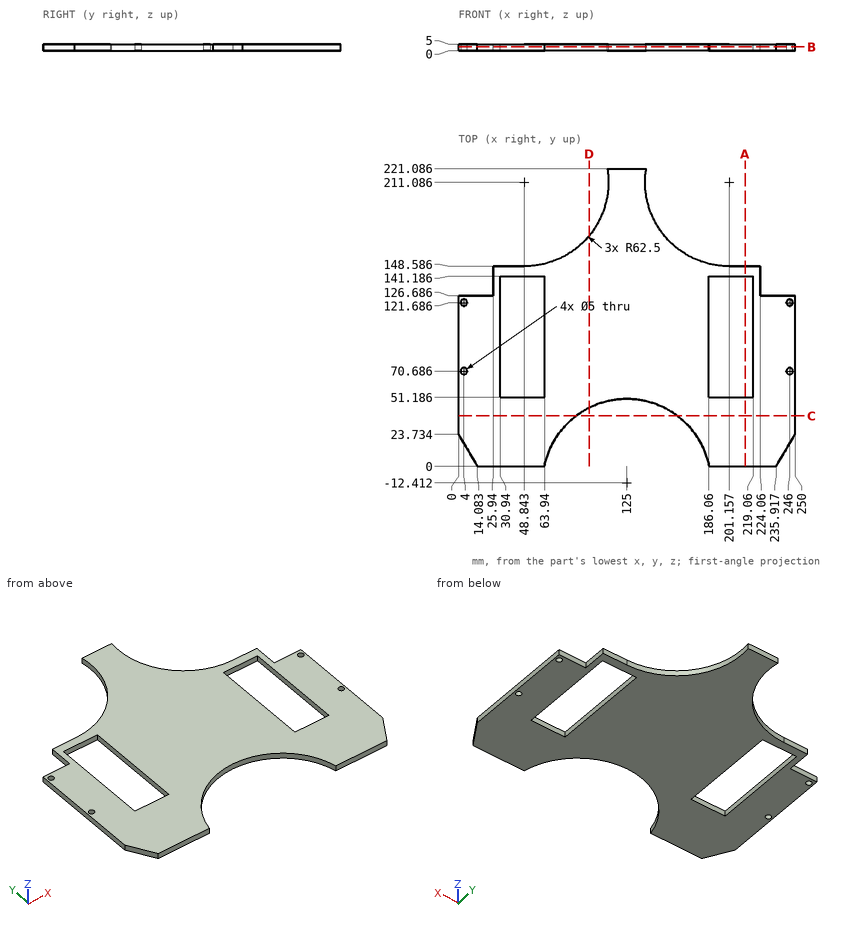
The figure shows three views and two pictorial views of one solid part (mm, origin at its lowest corner). Answer the questions. Coordinates: 2 decimals unless noted, no trailing zeros. Loops run counter-clockwise (first coordinate to the right, second up) from the corner with the lowest first, then second, coordinate; pieces in that order, holes last. Notation, with made-up numbers: (58.25, 70.25) - (94.25, 70.25) arc R17 ccw to (94.25, 95.25) - close; hole circle Ø7 at (-39.75, -33). An arc over 180 degrees is marked (long way). Answer in a Markdown table with one row per item.
Q1. Find section A-A on x = 213. Write down the section's boundary in (y, z) (1 decimal).
Here are the results:
| item | result |
|---|---|
| outline | (0, 0) - (51.2, 0) - (51.2, 5) - (0, 5) - close; (141.2, 0) - (148.6, 0) - (148.6, 5) - (141.2, 5) - close |
Q2. Find section C-C on y = 37.5. Write down the section's boundary in (x, z).
Here are the results:
| item | result |
|---|---|
| outline | (0, 0) - (87.38, 0) - (87.38, 5) - (0, 5) - close; (162.62, 0) - (250, 0) - (250, 5) - (162.62, 5) - close |
Q3. Straight lines are drawn through the part: line 1 along X through (y, z) = (65, 0.9); line 2 along X through (y, z) = (139.5, 2.8); line 3 along Y through (x, z) = (246, 2.1) (1 decimal). For each, find the intervals that lie inside material, in ascending order. Write a range as [from, to].
Here are the results:
| item | result |
|---|---|
| line 1 | x = [0, 30.94], [63.94, 186.06], [219.06, 250] |
| line 2 | x = [25.94, 30.94], [63.94, 186.06], [219.06, 224.06] |
| line 3 | y = [17, 68.2], [73.2, 119.2], [124.2, 126.7] |
Q4. Find section D-D on x = 97. Write down the section's boundary in (y, z) (1 decimal), plus the area to 3 significant figures.
Here are the results:
| item | result |
|---|---|
| outline | (43.5, 0) - (171.2, 0) - (171.2, 5) - (43.5, 5) - close |
| area | 639 mm^2 |
Q5. Find section B-B on z = 2.95. Write down the section's boundary in (x, y) (1 decimal).
Here are the results:
| item | result |
|---|---|
| outline | (0, 23.7) - (14.1, 0) - (63.7, 0) arc R62.5 cw to (186.3, 0) - (235.9, 0) - (250, 23.7) - (250, 126.7) - (224.1, 126.7) - (224.1, 148.6) - (201.2, 148.6) arc R62.5 cw to (139.5, 221.1) - (110.5, 221.1) arc R62.5 cw to (48.8, 148.6) - (25.9, 148.6) - (25.9, 126.7) - (0, 126.7) - close; hole circle Ø5 at (4, 70.7); hole circle Ø5 at (4, 121.7); hole (30.9, 51.2) - (63.9, 51.2) - (63.9, 141.2) - (30.9, 141.2) - close; hole (186.1, 51.2) - (219.1, 51.2) - (219.1, 141.2) - (186.1, 141.2) - close; hole circle Ø5 at (246, 70.7); hole circle Ø5 at (246, 121.7) |
Q6. Given P1, Ø1.5, axis at x = 196, z = 3, coming from the +Y side (1 decimal); P2, Ø1.5, axis at x = 101.5, z = 2.5, coming from the +Y side; P3, Ø3, axis at x = 62, z = 4, coming from the +Y side, each flat-ended and moving along its own axis, determine where each tip first touches the part or whether it passes through.
Here are the results:
| item | result |
|---|---|
| P1 | stops at y = 148.9 |
| P2 | stops at y = 178.62 |
| P3 | stops at y = 150.33 |
